Geometry check sheet. Reference: the model listing, model coordinates, mm. Face numbers are marked on the shaded views. A direction names the side the tool comes from. Coordinates: 2 decimals unless noted, no trailing zeros. Loops run counter-clockwise (first coordinate to the right, second up) from the corner with the lowest first, then second, coordinate; pieces in that order, holes last.
Autodesk Inventor part; units mm, degrees
ref_plane "YZ Plane" through (0, 0, 0) normal (1, 0, 0) x (0, 1, 0)
ref_plane "XZ Plane" through (0, 0, 0) normal (0, 1, 0) x (-1, 0, 0)
ref_plane "XY Plane" through (0, 0, 0) normal (0, 0, 1) x (1, 0, 0)
sketch "Sketch1" plane through (0, 0, 0) normal (0, 1, 0) x (-1, 0, 0)
  line L0 (-88.9, 44.45) -> (88.9, 44.45)
  line L1 (88.9, 44.45) -> (88.9, -44.45)
  line L2 (88.9, -44.45) -> (-88.9, -44.45)
  line L3 (-88.9, -44.45) -> (-88.9, 44.45)
  line L4 (-88.9, 44.45) -> (88.9, -44.45) construction
  line L5 (88.9, 44.45) -> (-88.9, -44.45) construction
  line L6 (-66.04, -8.89) -> (-15.24, -8.89)
  line L7 (-15.24, -8.89) -> (-15.24, -21.59)
  line L8 (-15.24, -21.59) -> (-66.04, -21.59)
  line L9 (-66.04, -21.59) -> (-66.04, -8.89)
  line L10 (-66.04, -8.89) -> (-15.24, -21.59) construction
  line L11 (-15.24, -8.89) -> (-66.04, -21.59) construction
  point P0 (0, 0)
  point P1 (-40.64, -15.24)
  dimension "d0" = 177.8
  dimension "d1" = 88.9
  dimension "d2" = 22.86
  dimension "d3" = 22.86
  dimension "d4" = 12.7
  dimension "d5" = 50.8
extrude "Extrusion1" add sketch "Sketch1" along normal blind 3.175 contours L0 L1 L2 L3 | L6 L7 L8 L9
extrude "Extrusion2" add sketch "Sketch1" against normal blind 15.24 contours L6 L7 L8 L9
sketch "Sketch2" plane through (0, 0, 0) normal (0, -1, 0) x (1, 0, 0)
  circle A0 centre (-79.375, 34.925) radius 3.175
  circle A1 centre (-79.375, -34.925) radius 3.175
  circle A2 centre (79.375, 34.925) radius 3.175
  circle A3 centre (79.375, -34.925) radius 3.175
  line L0 (88.9, 44.45) -> (-88.9, 44.45)
  line L1 (-88.9, 44.45) -> (-88.9, -44.45)
  line L2 (-88.9, -44.45) -> (88.9, -44.45)
  line L3 (88.9, -44.45) -> (88.9, 44.45)
  point P0 (0, 0)
  dimension "d11" = 9.525
  dimension "d13" = 9.525
  dimension "d14" = 6.35
  dimension "d15" = 9.525
  dimension "d16" = 9.525
equation "\"d11\" = d10"
equation "\"d13\" = d12"
equation "\"d15\" = d11"
equation "\"d16\" = d13"
equation "\"d12\" = d11"
properties part number "BackCover"
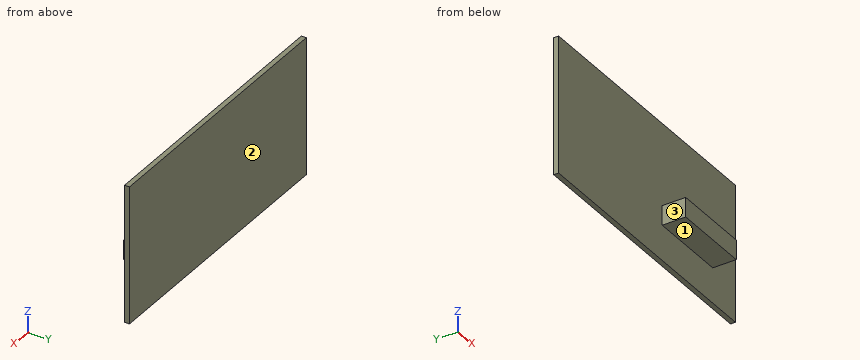
(1) Sectioned sample at C-C on z = -2.5. Record the cut outline in (x, y) (3 decimals).
Findings:
outline: (-88.9, 0) - (88.9, 0) - (88.9, 3.175) - (-88.9, 3.175) - close
(2) Scan lines: L1, parallel to Y at x = 2, z = 37 (3 decimals); L2, parallel to Z at x = 37.5, y = -13.75; L3, parallel to X at y = -6.25, z = -12. Record each from-to range of solid material in increasing order.
Findings:
L1: y = 0 to 3.175
L2: z = -21.59 to -8.89
L3: x = 15.24 to 66.04
(3) Sectioned sample at B-B on y = -13.5. Record the cut outline in (x, z).
Findings:
outline: (15.24, -21.59) - (66.04, -21.59) - (66.04, -8.89) - (15.24, -8.89) - close
(4) Gauge pin test, flat ends, axial feed: pin 1 Ø2 at (x, y) = (35, -1.5) entering from +Z; pin 2 Ø6 at (x, z) = (-66, 12) entering from -Y; pin 3 Ø10 at (y, z) = (-9, -14) entering from +X; pin 4 Ø4 at (y, z) = (-1, 19) entering from +X. Record the tip position at first contact, or that the pin passes through.
Findings:
pin 1: stops at z = -8.89
pin 2: stops at y = 0
pin 3: stops at x = 66.04
pin 4: stops at x = 88.9
(5) Access from +Z, -Z, +X, -X, +Y, -Y to the whole of each face (thin tool, end or side, straight path). Record for the marked faces 1, 2 and 3.
Findings:
face 1: -Z, +X, -X, -Y
face 2: +Z, -Z, +X, -X, +Y
face 3: +Z, -Z, -X, -Y
(6) Sectioned sample at A-A on x = 44.5. Record the cut outline in (y, z) (3 decimals), and give its area (3 significant figures).
Findings:
outline: (-15.24, -21.59) - (0, -21.59) - (0, -44.45) - (3.175, -44.45) - (3.175, 44.45) - (0, 44.45) - (0, -8.89) - (-15.24, -8.89) - close
area: 476 mm2
